The figure shows three views and two pictorial views of one solid part (mm, origin at its lowest corner). Answer the questions. A direction names the side the tool comes from. Round coordinates to 2 decimals unless told otherwise and drop trailing zeros. Order: outer loops, then holes, each group sorted by start corner. A loop starts at its lowest first (then second) coordinate and runs counter-clockwise, first axis right, second up. Notation, with made-up numbers: (-19.5, 9) - (8.5, 9) arc R4 ccw to (8.5, 14) - close; hole circle Ø1 at (76.25, -19). An arc over 180 degrees is marked (long way). Answer in a Markdown table with one row per item.
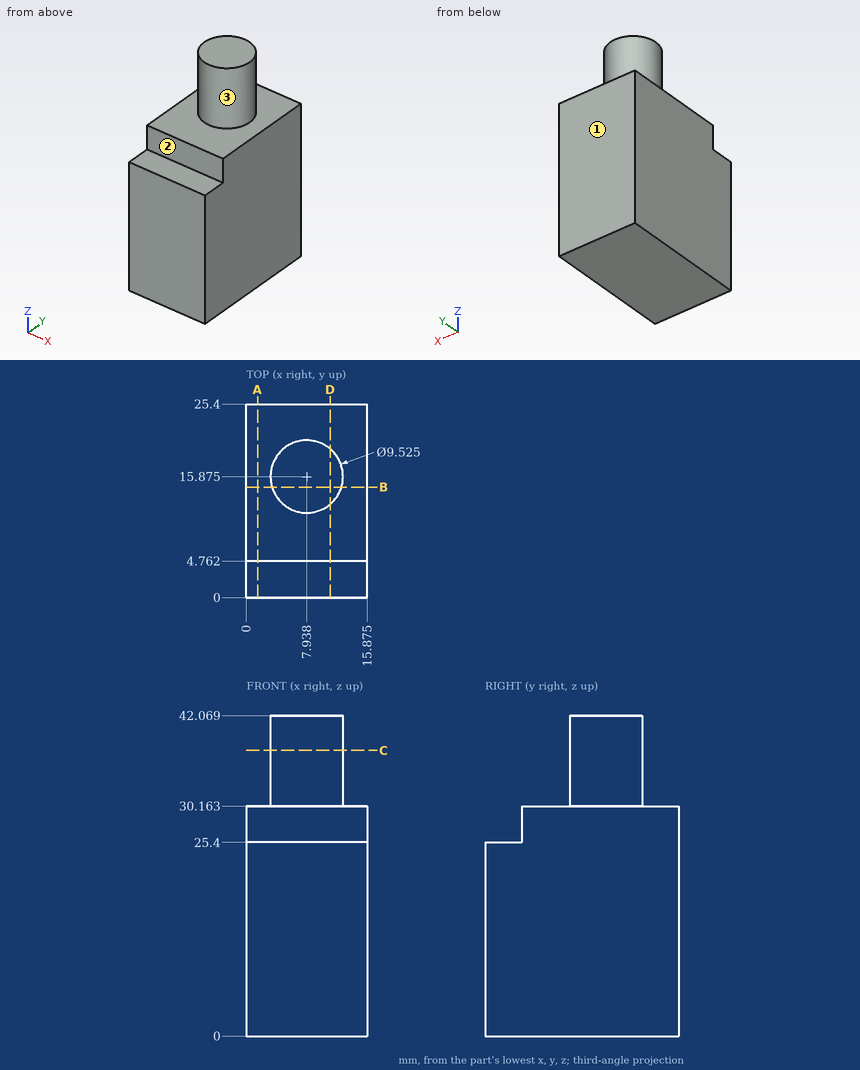
1) Find section B-B, the plane y = 14.5. Give the vertices of the cut face in (x, z) (1 decimal).
Filled in:
| item | result |
|---|---|
| outline | (0, 0) - (15.9, 0) - (15.9, 30.2) - (12.5, 30.2) - (12.5, 42.1) - (3.4, 42.1) - (3.4, 30.2) - (0, 30.2) - close |
2) Which of the six approach directions +Z, -Z, +X, -X, +Y, -Y give full straight-line access (tool end or side, diameter ignored) to the marked faces 1, 2 and 3?
Filled in:
| item | result |
|---|---|
| face 1 | +Z, -Z, +X, -X, +Y |
| face 2 | +Z, +X, -X, -Y |
| face 3 | +Z |
3) Find section A-A, the plane x = 1.5. Give the vertices of the cut face in (y, z).
Filled in:
| item | result |
|---|---|
| outline | (0, 0) - (25.4, 0) - (25.4, 30.16) - (4.76, 30.16) - (4.76, 25.4) - (0, 25.4) - close |
4) Find the intervals of material crossed by probe 1 along Z at (x, y) = (7.75, 7.5); probe 2 along Y at (x, z) = (8, 30); probe 3 along Y at (x, z) = (9.5, 38) (1 decimal), in increasing order. Write a range as from..to.
Filled in:
| item | result |
|---|---|
| probe 1 | z = 0..30.16 |
| probe 2 | y = 4.76..25.4 |
| probe 3 | y = 11.4..20.4 |
5) Each of these flat-tipped pins is pushed along its axis until it touches: pin 1 (4 mm diameter, centred on x = 9, z = 27.5, fed in from -Y); pin 2 (5 mm diameter, centred on x = 6.5, y = 3.5, fed in from +Z). Where does it stop, or does it pass through?
Filled in:
| item | result |
|---|---|
| pin 1 | stops at y = 4.76 |
| pin 2 | stops at z = 30.16 |
6) Find section D-D, the plane x = 11. Give the vertices of the cut face in (y, z), then the cut area to 3 significant figures.
Filled in:
| item | result |
|---|---|
| outline | (0, 0) - (25.4, 0) - (25.4, 30.16) - (19.52, 30.16) - (19.52, 42.07) - (12.23, 42.07) - (12.23, 30.16) - (4.76, 30.16) - (4.76, 25.4) - (0, 25.4) - close |
| area | 830 mm^2 |
7) Find section C-C, the plane z = 37.5. Give the vertices of the cut face in (x, y) (1 decimal).
Filled in:
| item | result |
|---|---|
| outline | circle Ø9.5 at (7.9, 15.9) |
